Source: CAD feature listing. Evaluate the final solid. Frame: model axes, mm. A direction names the side the tool comes from. Round coordinates to 2 decimals unless told otherwise and drop trailing zeros. Write each loop counter-clockwise with the first axis right and the second up, starting at its lowest first coordinate (ties: lowest second). Pieces come first, ordered by that corner, then holes. Notation, with made-up numbers: M 57.5,-2 L 95.5,-2 A36 ccw 95.5,34 Z; hole C 85,-18 d1. An arc over 180 degrees is marked long. Answer in a Markdown table with one row per item.
from build123d import *

# Parameters (mm, degrees)
F0_W     = 12.86
F0_H     = 12.86
F0_R     = 2.25
F0_R_2   = 19.05
F1_DEPTH = 6.8
F2_DEPTH = 1.6
F3_DEPTH = 88
F4_R     = 4.45
F5_R     = 2
F6_DEPTH = 10
F7_DEPTH = 24
F8_DEPTH = 103
F9_SIZE  = 0.3


with BuildPart() as f1:
    # F0 (on Front) → F1 (new body)
    with BuildSketch(Plane.XZ):
        with Locations((23.57, -23.57)):
            Rectangle(F0_W, F0_H)
        with Locations((23.57, -23.57)):
            Circle(F0_R, mode=Mode.SUBTRACT)
        Polygon((-17.14, -30), (17.14, -30), (17.14, -17.14), (30, -17.14), (30, 17.14), (17.14, 17.14), (17.14, 30), (-17.14, 30), (-17.14, 17.14), (-30, 17.14), (-30, -17.14), (-17.14, -17.14), align=None)
        Circle(F0_R_2, mode=Mode.SUBTRACT)
        with Locations((-23.57, -23.57)):
            Rectangle(F0_W, F0_H)
        with Locations((-23.57, -23.57)):
            Circle(F0_R, mode=Mode.SUBTRACT)
        with Locations((23.57, 23.57)):
            Rectangle(F0_W, F0_H)
        with Locations((23.57, 23.57)):
            Circle(F0_R, mode=Mode.SUBTRACT)
        with Locations((-23.57, 23.57)):
            Rectangle(F0_W, F0_H)
        with Locations((-23.57, 23.57)):
            Circle(F0_R, mode=Mode.SUBTRACT)
        Circle(F0_R_2)
        with BuildLine():
            ThreePointArc((-3.5, 1.9364916731), (1, 3.8729833462), (4, 0))
            ThreePointArc((4, 0), (1, -3.8729833462), (-3.5, -1.9364916731))
            ThreePointArc((-3.5, -1.9364916731), (-4, 0), (-3.5, 1.9364916731))
        make_face(mode=Mode.SUBTRACT)
    extrude(amount=-F1_DEPTH)

    # F0 (on Front) → F2 (join)
    with BuildSketch(Plane.XZ):
        Circle(F0_R_2)
        with BuildLine():
            ThreePointArc((-3.5, 1.9364916731), (1, 3.8729833462), (4, 0))
            ThreePointArc((4, 0), (1, -3.8729833462), (-3.5, -1.9364916731))
            ThreePointArc((-3.5, -1.9364916731), (-4, 0), (-3.5, 1.9364916731))
        make_face(mode=Mode.SUBTRACT)
    extrude(amount=F2_DEPTH)

    # F0 (on Front) → F3 (join)
    with BuildSketch(Plane.XZ):
        Polygon((-17.14, -30), (17.14, -30), (17.14, -17.14), (30, -17.14), (30, 17.14), (17.14, 17.14), (17.14, 30), (-17.14, 30), (-17.14, 17.14), (-30, 17.14), (-30, -17.14), (-17.14, -17.14), align=None)
        Circle(F0_R_2, mode=Mode.SUBTRACT)
        Circle(F0_R_2)
        with BuildLine():
            ThreePointArc((-3.5, 1.9364916731), (1, 3.8729833462), (4, 0))
            ThreePointArc((4, 0), (1, -3.8729833462), (-3.5, -1.9364916731))
            ThreePointArc((-3.5, -1.9364916731), (-4, 0), (-3.5, 1.9364916731))
        make_face(mode=Mode.SUBTRACT)
    extrude(amount=-F3_DEPTH)

    # F4
    f4_edges = [f1.edges().sort_by_distance(p)[0] for p in [
        (17.14, 47.4, 17.14),
        (17.14, 47.4, -17.14),
        (-17.14, 47.4, 17.14),
        (-17.14, 47.4, -17.14),
    ]]
    fillet(f4_edges, radius=F4_R)

    # F5
    f5_edges = [f1.edges().sort_by_distance(p)[0] for p in [
        (-30, 3.4, 30),
        (30, 3.4, 30),
        (-17.14, 47.4, 30),
        (-30, 47.4, 17.14),
        (17.14, 47.4, 30),
        (-30, 3.4, -30),
        (30, 3.4, -30),
        (30, 47.4, 17.14),
        (30, 47.4, -17.14),
        (17.14, 47.4, -30),
        (-17.14, 47.4, -30),
        (-30, 47.4, -17.14),
    ]]
    fillet(f5_edges, radius=F5_R)

    # F0 (on Front) → F6 (join)
    with BuildSketch(Plane.XZ):
        with BuildLine():
            Line((-3.5, -1.9364916731), (-3.5, 1.9364916731))
            ThreePointArc((-3.5, 1.9364916731), (-4, 0), (-3.5, -1.9364916731))
        make_face()
    extrude(amount=F6_DEPTH)

    # F0 (on Front) → F7 (join)
    with BuildSketch(Plane.XZ):
        with BuildLine():
            ThreePointArc((-3.5, -1.9364916731), (1, -3.8729833462), (4, 0))
            ThreePointArc((4, 0), (1, 3.8729833462), (-3.5, 1.9364916731))
            Line((-3.5, 1.9364916731), (-3.5, -1.9364916731))
        make_face()
    extrude(amount=F7_DEPTH)

    # F0 (on Front) → F8 (join)
    with BuildSketch(Plane.XZ):
        with BuildLine():
            ThreePointArc((-3.5, -1.9364916731), (1, -3.8729833462), (4, 0))
            ThreePointArc((4, 0), (1, 3.8729833462), (-3.5, 1.9364916731))
            Line((-3.5, 1.9364916731), (-3.5, -1.9364916731))
        make_face()
    extrude(amount=-F8_DEPTH)

    # F9
    f9_edges = [f1.edges().sort_by_distance(p)[0] for p in [
        (4, -24, 0),
        (-3.5, -24, 0),
        (-19.05, -1.6, 0),
    ]]
    chamfer(f9_edges, length=F9_SIZE)


solid = f1.part
Q1. Access query for faces 1 (the cylindrical face through (-18.409, 47.968, 18.478)), 2 (the flat face through (-17.14, 47, -25)), 3 (the flat face through (-3.5, -17, 0)). Directions: +Z, -Z, +X, -X, +Y, -Y. A direction counts if a zero-diameter tool reaches every point of the face in a straight line with its end or side. Return the directions, or none.
Solutions:
| item | result |
|---|---|
| face 1 | +Z, -X, +Y |
| face 2 | -Z, -X, +Y |
| face 3 | +Z, -Z, -X, -Y |
Q2. Section D-D (x = 0). Return loops of the section in (y, z), and give its area (3 significant figures).
Solutions:
| item | result |
|---|---|
| outline | M -24,-3.7 L -23.7,-4 L -1.6,-4 L -1.6,-18.75 L -1.3,-19.05 L 0,-19.05 L 0,-30 L 88,-30 L 88,-4 L 103,-4 L 103,4 L 88,4 L 88,30 L 0,30 L 0,19.05 L -1.3,19.05 L -1.6,18.75 L -1.6,4 L -23.7,4 L -24,3.7 Z |
| area | 5,640 mm2 |
Q3. Section B-B (x = 23.57). Return loops of the section in (y, z), and give its area (3 significant figures).
Solutions:
| item | result |
|---|---|
| outline | M 0,-30 L 6.8,-30 L 6.8,-25.82 L 0,-25.82 Z; M 0,-21.32 L 6.8,-21.32 L 6.8,-17.14 L 88,-17.14 L 88,17.14 L 6.8,17.14 L 6.8,21.32 L 0,21.32 Z; M 0,25.82 L 6.8,25.82 L 6.8,30 L 0,30 Z |
| area | 3,130 mm2 |
Q4. Material intervals for probe 1 along Z at (x, y) = (-23.57, 2); probe 2 along Z at (x, y) = (23, 3), sorted ascending.
Solutions:
| item | result |
|---|---|
| probe 1 | z = -30 to -25.82, -21.32 to 21.32, 25.82 to 30 |
| probe 2 | z = -30 to -25.75, -21.39 to 21.39, 25.75 to 30 |
Q5. Contact query for flat-ended pins moving along their axis: pin 1 Ø3 at (y, z) = (50.5, -24.5) entering from -X; pin 2 Ø3 at (x, y) = (-23.5, 49.5) entering from +Z; pin 3 Ø1.5 at (y, z) = (15.5, -16.5) entering from +X; pin 4 Ø4 at (x, z) = (-23.57, -23.57) entering from +Y. Output: stop coordinate, or through.
Solutions:
| item | result |
|---|---|
| pin 1 | stops at x = -17.14 |
| pin 2 | stops at z = 17.14 |
| pin 3 | stops at x = 29.9 |
| pin 4 | passes through |
Q6. Section C-C (y = 49.5). Return loops of the section in (x, z).
Solutions:
| item | result |
|---|---|
| outline | M -30,-15.14 A2 ccw -28,-17.14 L -21.59,-17.14 A4.45 cw -17.14,-21.59 L -17.14,-28 A2 ccw -15.14,-30 L 15.14,-30 A2 ccw 17.14,-28 L 17.14,-21.59 A4.45 cw 21.59,-17.14 L 28,-17.14 A2 ccw 30,-15.14 L 30,15.14 A2 ccw 28,17.14 L 21.59,17.14 A4.45 cw 17.14,21.59 L 17.14,28 A2 ccw 15.14,30 L -15.14,30 A2 ccw -17.14,28 L -17.14,21.59 A4.45 cw -21.59,17.14 L -28,17.14 A2 ccw -30,15.14 Z; hole M -3.5,-1.94 L -3.5,1.94 A4 ccw Z |
Q7. Section A-A (z = 23.57). Return loops of the section in (x, y), and give its area (3 significant figures).
Solutions:
| item | result |
|---|---|
| outline | M -30,0 L -25.82,0 L -25.82,6.8 L -30,6.8 Z; M -21.32,0 L 21.32,0 L 21.32,6.8 L 17.14,6.8 L 17.14,88 L -17.14,88 L -17.14,6.8 L -21.32,6.8 Z; M 25.82,0 L 30,0 L 30,6.8 L 25.82,6.8 Z |
| area | 3,130 mm2 |
Q8. Pull-direction query (X, two-part tool) for faces 4 (the flat face through (17.14, 47, -25)), 5 (the cylindrical face through (21.91, 3.35, 25.09)), 6 (the flat face through (24, 6.8, 26)); classes: pulls with the +X half, pulls with the -X half, needs draft (parallel to the pull), parting line crosses it, or undercut.
Solutions:
| item | result |
|---|---|
| face 4 | pulls with the +X half |
| face 5 | undercut |
| face 6 | needs draft |
